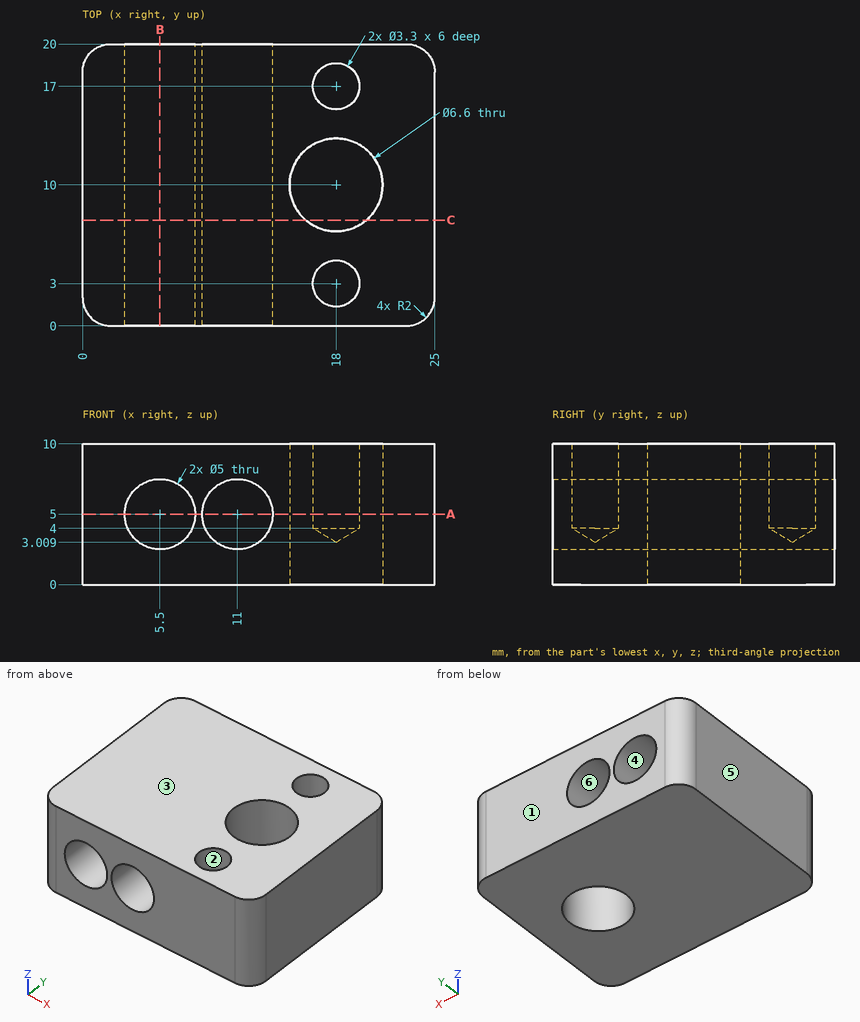
Geometry check sheet. Reference: drawing and pictorial views, mm from the part's lowest x, y, z. A direction names the side the tool comes from. Round coordinates to 2 decimals unless told otherwise and drop trailing zeros. Loops run counter-clockwise (first coordinate to the right, second up) from the corner with the lowest first, then second, coordinate; pieces in that order, holes last. Notation, with made-up numbers: (31, 21) - (85, 21) arc R28 cw to (85, 42) - close; hole circle Ø7 at (-17, 49.25). An arc over 180 degrees is marked (long way). One line per question, with ' | ' between items. Start each with the question number.
1. Draft check along X on the marked faces 3, 4, 5 and 6. Enter one of: released by +X, released by -X, zero draft, split by the parting line, or undercut.
2. Cross-section at C-C on y = 7.5. Record the cut outline in (x, z).
3. Tool access check on the marked faces 1 and 2. Record the directions out of +Z, -Z, +X, -X, +Y, -Y that give a thin tool (end or side, any length) a straight path to the whole face; none if there is none.
4. Depth check by flat-ended pin: pin 1 (5.5 mm diameter, centred on x = 18, y = 10, fed in from -Z); pin 2 (3 mm diameter, centred on x = 18, y = 3, fed in from +Z). Enter the tip coordinate at first touch or a pass-through.
5. Cross-section at A-A on z = 5. Record the cut outline in (x, y), then the cut area to 3 significant figures.
6. Scan lines: line 1 (Y direction, x = 18, z = 6); line 2 (X direction, y = 17, z = 7.95); line 3 (X direction, y = 19.25, z = 4). Record each from-to range of solid material in increasing order. Write a range as [from, to].
7. Cross-section at B-B on x = 5.5. Record the cut outline in (y, z).
Taken from the geometry:
1) face 3: zero draft | face 4: undercut | face 5: released by -X | face 6: undercut
2) outline: (0, 0) - (15.85, 0) - (15.85, 10) - (0, 10) - close; (20.15, 0) - (25, 0) - (25, 10) - (20.15, 10) - close; hole circle Ø5 at (5.5, 5); hole circle Ø5 at (11, 5)
3) face 1: +Z, -Z, +X, -X, +Y | face 2: +Z
4) pin 1: through | pin 2: z = 3.91
5) outline: (0, 2) arc R2 ccw to (2, 0) - (3, 0) - (3, 20) - (2, 20) arc R2 ccw to (0, 18) - close; (8, 0) - (8.5, 0) - (8.5, 20) - (8, 20) - close; (13.5, 0) - (23, 0) arc R2 ccw to (25, 2) - (25, 18) arc R2 ccw to (23, 20) - (13.5, 20) - close; hole circle Ø6.6 at (18, 10); hole circle Ø3.3 at (18, 3); hole circle Ø3.3 at (18, 17) | area: 245 mm²
6) line 1: [0, 1.35], [4.65, 6.7], [13.3, 15.35], [18.65, 20] | line 2: [0, 16.35], [19.65, 25] | line 3: [0.44, 3.21], [7.79, 8.71], [13.29, 24.56]
7) outline: (0, 0) - (20, 0) - (20, 2.5) - (0, 2.5) - close; (0, 7.5) - (20, 7.5) - (20, 10) - (0, 10) - close
